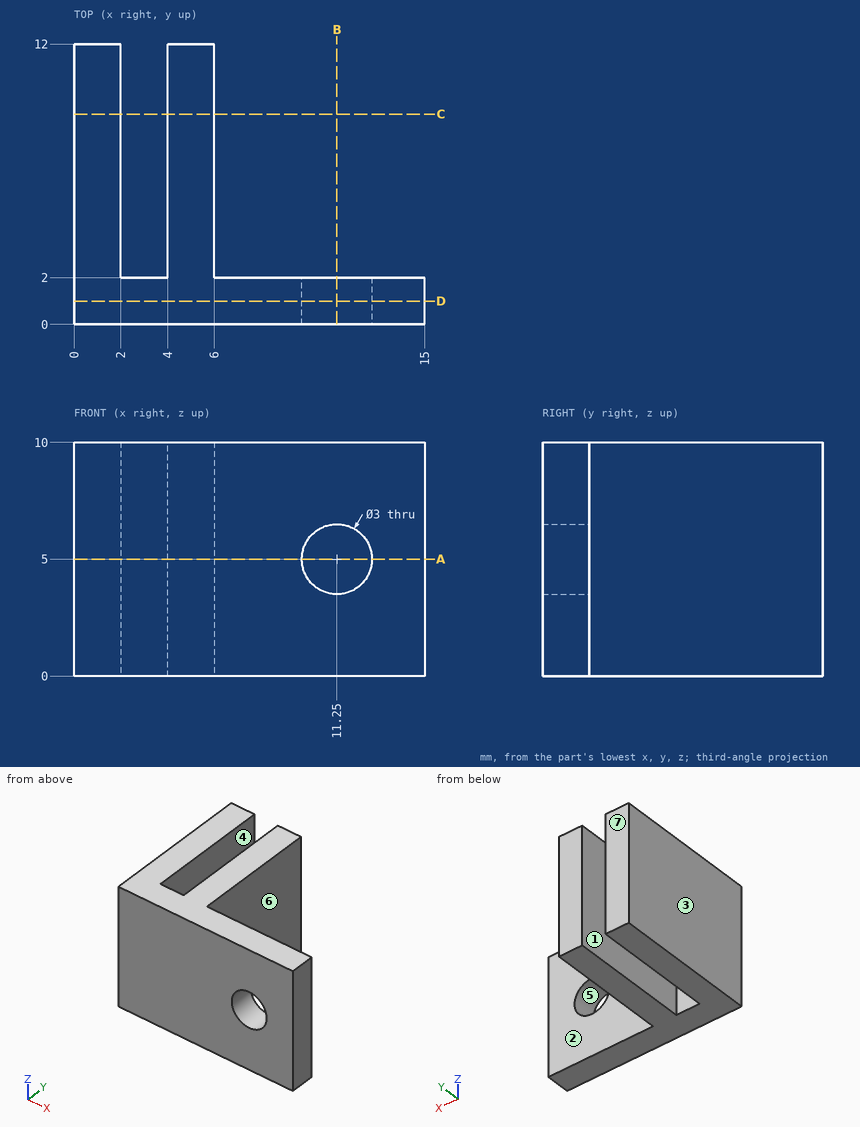
Check sheet for the drawn part. Datum: minimum x, y, z corner. Units: mm. A direction names the side the tool comes from. Round coordinates to 2 decimals unless told otherwise and drop trailing zeros. Write each loop counter-clockwise with the first axis right and the second up, starting at its lowest first coordinate (ties: lowest second). Pieces come first, ordered by that corner, then holes. Notation, with made-up numbers: (10.5, 72.5) -> (39.5, 72.5) arc R18 ccw to (39.5, 83.5) -> close; hole circle Ø4 at (39.25, 81.5). An arc over 180 degrees is marked (long way). Put each result on its own line as item: value.
(1) Sectioned sample at D-D (y = 1). Enter the section's corners in (x, z), plus the area to 3 significant figures.
Values found:
outline: (0, 0) -> (15, 0) -> (15, 10) -> (0, 10) -> close; hole circle Ø3 at (11.25, 5)
area: 143 mm^2
(2) Sectioned sample at C-C (y = 9). Enter the section's corners in (x, z), plus the area to 3 significant figures.
Values found:
outline: (0, 0) -> (2, 0) -> (2, 10) -> (0, 10) -> close; (4, 0) -> (6, 0) -> (6, 10) -> (4, 10) -> close
area: 40.0 mm^2
(3) Go/stop test with flat-tipped pins: pin 1 Ø3 at (x, y) = (4.5, 5.5) entering from -Z; pin 2 Ø5 at (y, z) = (8.5, 3.5) entering from +X; pin 3 Ø1.5 at (x, y) = (3, 4.5) entering from -Z; pin 4 Ø0.6 at (x, z) = (3, 5) entering from +Y. Record where each tip stops, or that it passes through.
Values found:
pin 1: stops at z = 0
pin 2: stops at x = 6
pin 3: passes through
pin 4: stops at y = 2
(4) Mould release check, pull along X, two halves, no side actions. Record for the marked faces 4, 5, 6 and 7: released by +X, released by -X, zero draft, split by the parting line, or undercut.
Values found:
face 4: undercut
face 5: undercut
face 6: released by +X
face 7: zero draft
(5) Sectioned sample at B-B (x = 11.25). Enter the section's corners in (y, z).
Values found:
outline: (0, 0) -> (2, 0) -> (2, 3.5) -> (0, 3.5) -> close; (0, 6.5) -> (2, 6.5) -> (2, 10) -> (0, 10) -> close
(6) Material ranges on line 1 (X direction, y = 5, z = 5.25); line 2 (X direction, y = 1.35, z = 5); line 3 (Z direction, x = 11.25, y = 1.45), recorded low to high.
Values found:
line 1: x = 0 to 2, 4 to 6
line 2: x = 0 to 9.75, 12.75 to 15
line 3: z = 0 to 3.5, 6.5 to 10
(7) Sectioned sample at A-A (z = 5). Enter the section's corners in (x, y).
Values found:
outline: (0, 0) -> (9.75, 0) -> (9.75, 2) -> (6, 2) -> (6, 12) -> (4, 12) -> (4, 2) -> (2, 2) -> (2, 12) -> (0, 12) -> close; (12.75, 0) -> (15, 0) -> (15, 2) -> (12.75, 2) -> close
(8) Tool access check on the marked faces 1, 2 and 3. Record the directions out of +Z, -Z, +X, -X, +Y, -Y that give a thin tool (end or side, any length) a straight path to the whole face; none if there is none.
Values found:
face 1: +Z, -Z, +Y
face 2: +Z, -Z, +X, +Y
face 3: +Z, -Z, -X, +Y, -Y
